Check sheet for the drawn part. Datum: minimum x, y, z corner. Units: mm. Coordinates: 2 decimals unless noted, no trailing zeros. Write each loop counter-clockwise with the first axis right and the second up, starting at its lowest first coordinate (ties: lowest second). Pieces come first, ordered by that corner, then holes. Notation, with made-up numbers: M -9.5,-37.75 L 45.5,-37.75 A15 cw 45.5,-33.75 Z; hole C 74.5,87 d9. An arc over 180 degrees is marked long. Answer as CSV lines item,"result".
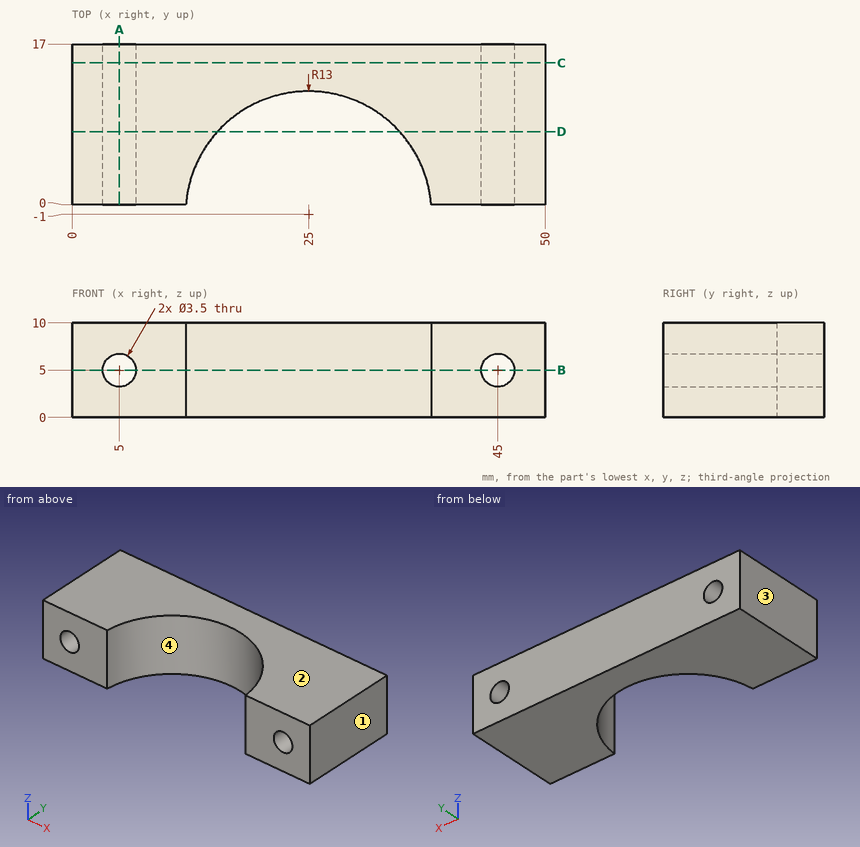
1) Section check C-C, the plane y = 15. Record the boundary of the cut face in (x, z).
Answer key:
outline,"M 0,0 L 50,0 L 50,10 L 0,10 Z; hole C 5,5 d3.5; hole C 45,5 d3.5"
2) Section check B-B, the plane z = 5. Record the boundary of the cut face in (x, y).
Answer key:
outline,"M 0,0 L 3.25,0 L 3.25,17 L 0,17 Z; M 6.75,0 L 12.04,0 A13 cw 37.96,0 L 43.25,0 L 43.25,17 L 6.75,17 Z; M 46.75,0 L 50,0 L 50,17 L 46.75,17 Z"
3) Section check D-D, the plane y = 7.75. Record the boundary of the cut face in (x, z), plus the area to 3 significant figures.
Answer key:
outline,"M 0,0 L 15.39,0 L 15.39,10 L 0,10 Z; M 34.61,0 L 50,0 L 50,10 L 34.61,10 Z; hole C 5,5 d3.5; hole C 45,5 d3.5"
area,"288 mm2"
4) Section check A-A, the plane x = 5. Record the boundary of the cut face in (y, z).
Answer key:
outline,"M 0,0 L 17,0 L 17,3.25 L 0,3.25 Z; M 0,6.75 L 17,6.75 L 17,10 L 0,10 Z"
5) Mould release check, pull along X, two halves, no side actions. Record for the marked faces 1, 2, 3 and 4: pulls with the +X half, pulls with the -X half, needs draft (parallel to the pull), parting line crosses it, or undercut.
Answer key:
face 1,"pulls with the +X half"
face 2,"needs draft"
face 3,"pulls with the -X half"
face 4,"undercut"
6) Thickness scan on line 1 along X through (y, z) = (6.5, 6.5); line 2 along Z through (x, y) = (5, 3.5); line 3 along X through (y, z) = (8.5, 5). Record the ranges inside material, lowest first.
Answer key:
line 1,"x = 0 to 4.1, 5.9 to 14.38, 35.62 to 44.1, 45.9 to 50"
line 2,"z = 0 to 3.25, 6.75 to 10"
line 3,"x = 0 to 3.25, 6.75 to 16.13, 33.87 to 43.25, 46.75 to 50"
